from build123d import *

# Parameters (mm, degrees)
F0_R      = 15
F1_DEPTH  = 12
F3_DEPTH  = 12.001
F4_R      = 15
F5_DEPTH  = 0.75
F6_R      = 9
F7_DEPTH  = 15.751
F9_R      = 2.5
F10_DEPTH = 12
F11_W     = 1.5
F11_H     = 12
F12_REACH = 42.0943866224
F13_W     = 1.5
F13_H     = 12
F14_DEPTH = 8


with BuildPart() as f1:
    # F0 (on Top) → F1 (new body)
    with BuildSketch(Plane.XY):
        Circle(F0_R)
    extrude(amount=F1_DEPTH)

    # F2 (on face) → F3 (cut, through all)
    with BuildSketch(Plane.XY.offset(12)):
        Polygon((7, -4.0414518843), (7, 4.0414518843), (0, 8.0829037687), (-7, 4.0414518843), (-7, -4.0414518843), (0, -8.0829037687), align=None)
    extrude(amount=-F3_DEPTH, mode=Mode.SUBTRACT)

    # F9 (on offset) → F10 (cut)
    with BuildSketch(Plane.XZ.offset(15)):
        with Locations((0, 6)):
            Circle(F9_R)
    extrude(amount=-F10_DEPTH, mode=Mode.SUBTRACT)



with BuildPart() as f5:
    # F4 (on Front) → F5 (new body, symmetric)
    with BuildSketch(Plane.XZ):
        with Locations((-36, 6)):
            Circle(F4_R)
    extrude(amount=F5_DEPTH, both=True)

    # F6 (on face) → F7 (cut, through all)
    with BuildSketch(Plane.XZ.offset(0.75)):
        with Locations((-36, 6)):
            Circle(F6_R)
    extrude(amount=-F7_DEPTH, mode=Mode.SUBTRACT)



with BuildPart() as f5b:
    # F4 (on Front) → F5, piece 2 (new body, symmetric)
    with BuildSketch(Plane.XZ):
        Polygon((-21, 0), (-15, 0), (-15, 12), (-21, 12), (-21, 6), align=None)
    extrude(amount=F5_DEPTH, both=True)


with BuildPart() as f5_1:
    add(f5.part)

    add(f5b.part)  # F12 merges F5b
    f12_end = f5_1.faces().sort_by_distance((-45, 0, 6))[0]
    # F11 (on face) → F12 (join, up to a face of the model that its end follows)
    with BuildSketch(Plane(origin=(-21, 0, 0), x_dir=(0, -1, 0), z_dir=(-1, 0, 0))):
        with Locations((0, 6)):
            Rectangle(F11_W, F11_H)
    f12_long = extrude(amount=F12_REACH, mode=Mode.PRIVATE)
    add(split(f12_long, bisect_by=f12_end, keep=Keep.ALL, mode=Mode.PRIVATE).solids().sort_by_distance((-21, 0, 6))[0])


with BuildPart() as f1_1:
    add(f1.part)

    add(f5_1.part)  # F14 merges F5
    # F13 (on face) → F14 (join, through all)
    with BuildSketch(Plane.YZ.offset(-15)):
        with Locations((0, 6)):
            Rectangle(F13_W, F13_H)
    extrude(amount=F14_DEPTH)


solid = f1_1.part
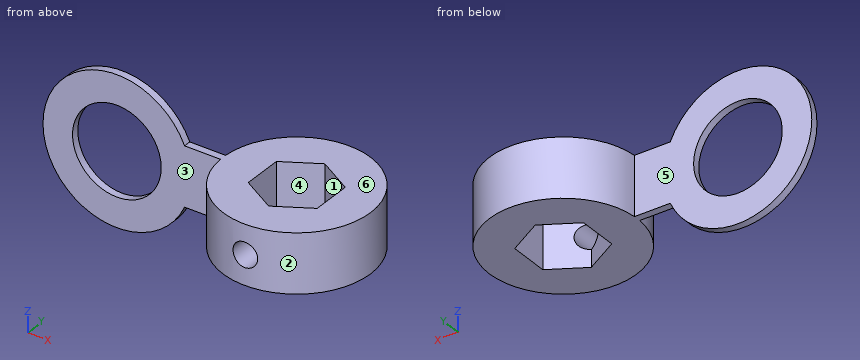
Geometry check sheet. Reference: the model listing, model coordinates, mm. Face numbers are marked on the shaded views. A direction names the side the tool comes from. Coordinates: 2 decimals unless noted, no trailing zeros. Order: outer loops, then holes, each group sorted by start corner. A loop starts at its lowest first (then second) coordinate and runs counter-clockwise, first axis right, second up. Notation, with made-up numbers: (82, 37.5) - (113, 37.5) arc R35 ccw to (113, 71.5) - close; hole circle Ø9 at (65, -39). An arc over 180 degrees is marked (long way). One line per item, written item: value.
(1) Depth check by flat-ended pin: pin 1 Ø6.5 at (y, z) = (-2, 8) entering from +X; pin 2 Ø12 at (x, y) = (8, -1.5) entering from +Z; pin 3 Ø4 at (y, z) = (10.5, 6) entering from -X; pin 4 Ø10 at (x, z) = (-31.5, 2) entering from -Y. Enter the tip coordinate at first touch or a pass-through.
Data:
pin 1: stops at x = 15
pin 2: stops at z = 12
pin 3: stops at x = -12.36
pin 4: stops at y = -0.75
(2) Sectioned sample at D-D (x = -11). Enter the section's corners in (y, z), and give its area (3 significant figures).
Data:
outline: (-10.2, 0) - (10.2, 0) - (10.2, 12) - (-10.2, 12) - close
area: 245 mm^2
(3) Thickness scan on probe 1 along Z at (x, y) = (-36, 0.1); probe 2 along Z at (x, y) = (0, -11.25); probe 3 along X at (y, z) = (0, 10.25). Record the ranges inside material, lowest first. Write a range as from..to.
Data:
probe 1: z = -9..-3, 15..21
probe 2: z = 0..3.5, 8.5..12
probe 3: x = -50.39..-43.93, -28.07..-7, 7..15
(4) Sectioned sample at A-A (y = 0). Enter the section's corners in (x, z), and give its area (3 significant figures).
Data:
outline: (-22.25, 0) - (-7, 0) - (-7, 12) - (-22.25, 12) arc R15 ccw (long way) to start; (7, 0) - (15, 0) - (15, 12) - (7, 12) - close; hole circle Ø18 at (-36, 6)
area: 721 mm^2
(5) Sectioned sample at B-B (x = -36). Enter the section's corners in (y, z), and give its area (3 significant figures).
Data:
outline: (-0.75, -9) - (0.75, -9) - (0.75, -3) - (-0.75, -3) - close; (-0.75, 15) - (0.75, 15) - (0.75, 21) - (-0.75, 21) - close
area: 18.0 mm^2
(6) Release check for a two-part mould opening along X. For the marked faces 1, 2 and 3 record: +X half, -X half, draft (parallel to the pull), parting line (faces both ways), or undercut.
Data:
face 1: undercut
face 2: parting line
face 3: draft
(7) Sectioned sample at C-C (y = -10.5). Enter the section's corners in (x, z).
Data:
outline: (-10.71, 0) - (10.71, 0) - (10.71, 12) - (-10.71, 12) - close; hole circle Ø5 at (0, 6)
(8) Access from +Z, -Z, +X, -X, +Y, -Y to the whole of each face (thin tool, end or side, straight path). Record for the marked faces 4, 5 and 6.
Data:
face 4: +Z, -Z
face 5: +Z, -Z, -X, +Y
face 6: +Z, +X, +Y, -Y
